Verification items for the finished model (mm, model axes). A direction names the side the tool comes from. Give positions to 0.01 mm unless a question says otherwise; leave off trailing zeros. Order: outer loops, then holes, each group sorted by start corner. A loop starts at its lowest first (then second) coordinate and runs counter-clockwise, first axis right, second up. Notation, with made-up numbers: (55.5, 84) - (100.5, 84) arc R31 ccw to (100.5, 123) - close; hole circle Ø8 at (-39.5, 63.5). An arc over 180 degrees is marked (long way). Answer as a JSON object with one key per item and string values.
```python
from build123d import *

# Parameters (mm, degrees)
SKETCH_1_R          = 7.6
EXTRUDE_1_DEPTH     = 450
SKETCH_2_R          = 7.6
SKETCH_2_R_2        = 4
CUT_EXTRUDE_1_DEPTH = 26
SKETCH_3_R          = 7.6
SKETCH_3_R_2        = 4
CUT_EXTRUDE_2_DEPTH = 38


with BuildPart() as part:
    # Эскиз1 → Бобышка-Вытянуть1 (new body)
    with BuildSketch(Plane(origin=(0, 0, 0), x_dir=(1, 0, 0), z_dir=(0, 1, 0))):
        Circle(SKETCH_1_R)
    extrude(amount=EXTRUDE_1_DEPTH)

    # Эскиз2 → Вырез-Вытянуть1 (cut)
    with BuildSketch(Plane(origin=(0, 450, 0), x_dir=(1, 0, 0), z_dir=(0, 1, 0))):
        Circle(SKETCH_2_R)
        Circle(SKETCH_2_R_2, mode=Mode.SUBTRACT)
    extrude(amount=-CUT_EXTRUDE_1_DEPTH, mode=Mode.SUBTRACT)

    # Эскиз3 → Вырез-Вытянуть2 (cut)
    with BuildSketch(Plane.XZ):
        Circle(SKETCH_3_R)
        Circle(SKETCH_3_R_2, mode=Mode.SUBTRACT)
    extrude(amount=-CUT_EXTRUDE_2_DEPTH, mode=Mode.SUBTRACT)


solid = part.part
```
(1) Section check B-B (x = 0). Record the cut outline in (y, z), then the cut area to 3 significant figures.
Computed values:
{"outline": "(0, -4) - (38, -4) - (38, -7.6) - (424, -7.6) - (424, -4) - (450, -4) - (450, 4) - (424, 4) - (424, 7.6) - (38, 7.6) - (38, 4) - (0, 4) - close", "area": "6,380 mm²"}
(2) Access from +Z, -Z, +X, -X, +Y, -Y to the whole of each face (thin tool, end or side, straight path). Record for faces 1 (the cylindrical face through (-7.593, 228.298, -0.334)), 2 (the flat face through (3, 424, 3)), 3 (the cylindrical face through (-0.867, 18.734, -3.905)).
Computed values:
{"face 1": "+Y, -Y", "face 2": "+Y", "face 3": "-Y"}
(3) Material ranges on line 1 along Y through (x, z) = (4.25, -5.25); line 2 along Z through (x, y) = (-6.5, 292.5); line 3 along Z through (x, y) = (-1, 236), recorded low to high. Write a range as [from, to].
Computed values:
{"line 1": "y = [38, 424]", "line 2": "z = [-3.94, 3.94]", "line 3": "z = [-7.53, 7.53]"}
(4) Section check A-A (z = 0). Record the cut outline in (x, y), then the cut area to 3 significant figures.
Computed values:
{"outline": "(-7.6, 38) - (-4, 38) - (-4, 0) - (4, 0) - (4, 38) - (7.6, 38) - (7.6, 424) - (4, 424) - (4, 450) - (-4, 450) - (-4, 424) - (-7.6, 424) - close", "area": "6,380 mm²"}
(5) Gauge pin test, flat ends, axial feed: pin 1 Ø1 at (x, z) = (3, 4) entering from +Y; pin 2 Ø1 at (y, z) = (130.5, 1.5) entering from +X; pin 3 Ø6 at (y, z) = (195, 5.5) entering from +X. Record the tip position at first contact, or that the pin passes through.
Computed values:
{"pin 1": "stops at y = 424", "pin 2": "stops at x = 7.53", "pin 3": "stops at x = 7.18"}
(6) Section check C-C (y = 145). Record the cut outline in (x, z).
Computed values:
{"outline": "circle Ø15.2 at (0, 0)"}
